```python
from build123d import *

# Parameters (mm, degrees)
F0_R     = 37
F1_DEPTH = 10
F2_R     = 37
F3_DEPTH = 75
F4_R     = 37
F4_R_2   = 30
F4_W     = 13
F4_H     = 13
F5_DEPTH = 10


with BuildPart() as f1:
    # F0 (on Top) → F1 (new body)
    with BuildSketch(Plane.XY):
        Circle(F0_R)
        with BuildLine():
            ThreePointArc((32.403703492, 2.5), (32.47591695, 1.250926958), (32.5, 0))
            ThreePointArc((32.5, 0), (32.47591695, -1.250926958), (32.403703492, -2.5))
            ThreePointArc((32.403703492, -2.5), (22.9809703886, -22.9809703886), (2.5, -32.403703492))
            ThreePointArc((2.5, -32.403703492), (0, -32.5), (-2.5, -32.403703492))
            ThreePointArc((-2.5, -32.403703492), (-22.9809703886, -22.9809703886), (-32.403703492, -2.5))
            ThreePointArc((-32.403703492, -2.5), (-32.5, 0), (-32.403703492, 2.5))
            ThreePointArc((-32.403703492, 2.5), (-22.9809703886, 22.9809703886), (-2.5, 32.403703492))
            ThreePointArc((-2.5, 32.403703492), (0, 32.5), (2.5, 32.403703492))
            ThreePointArc((2.5, 32.403703492), (22.9809703886, 22.9809703886), (32.403703492, 2.5))
        make_face(mode=Mode.SUBTRACT)
        with BuildLine():
            Line((2.5, 29.5), (2.5, 32.403703492))
            ThreePointArc((2.5, 32.403703492), (0, 32.5), (-2.5, 32.403703492))
            Line((-2.5, 32.403703492), (-2.5, 29.5))
            Line((-2.5, 29.5), (2.5, 29.5))
        make_face()
        with BuildLine():
            ThreePointArc((32.403703492, -2.5), (32.47591695, -1.250926958), (32.5, 0))
            ThreePointArc((32.5, 0), (32.47591695, 1.250926958), (32.403703492, 2.5))
            Line((32.403703492, 2.5), (29.5, 2.5))
            Line((29.5, 2.5), (29.5, -2.5))
            Line((29.5, -2.5), (32.403703492, -2.5))
        make_face()
        with BuildLine():
            ThreePointArc((-2.5, -32.403703492), (0, -32.5), (2.5, -32.403703492))
            Line((2.5, -32.403703492), (2.5, -29.5))
            Line((2.5, -29.5), (-2.5, -29.5))
            Line((-2.5, -29.5), (-2.5, -32.403703492))
        make_face()
        with BuildLine():
            Line((-29.5, 2.5), (-32.403703492, 2.5))
            ThreePointArc((-32.403703492, 2.5), (-32.5, 0), (-32.403703492, -2.5))
            Line((-32.403703492, -2.5), (-29.5, -2.5))
            Line((-29.5, -2.5), (-29.5, 2.5))
        make_face()
    extrude(amount=-F1_DEPTH)

    # F2 (on face) → F3 (join)
    with BuildSketch(Plane(origin=(0, 0, -10), x_dir=(1, 0, 0), z_dir=(0, 0, -1))):
        Circle(F2_R)
        with BuildLine():
            ThreePointArc((29.8956518578, 2.5), (29.9739016123, 1.2510883797), (30, 0))
            ThreePointArc((30, 0), (29.9739016123, -1.2510883797), (29.8956518578, -2.5))
            Line((29.8956518578, -2.5), (32.403703492, -2.5))
            ThreePointArc((32.403703492, -2.5), (22.9809703886, -22.9809703886), (2.5, -32.403703492))
            Line((2.5, -32.403703492), (2.5, -29.8956518578))
            ThreePointArc((2.5, -29.8956518578), (0, -30), (-2.5, -29.8956518578))
            Line((-2.5, -29.8956518578), (-2.5, -32.403703492))
            ThreePointArc((-2.5, -32.403703492), (-22.9809703886, -22.9809703886), (-32.403703492, -2.5))
            Line((-32.403703492, -2.5), (-29.8956518578, -2.5))
            ThreePointArc((-29.8956518578, -2.5), (-30, 0), (-29.8956518578, 2.5))
            Line((-29.8956518578, 2.5), (-32.403703492, 2.5))
            ThreePointArc((-32.403703492, 2.5), (-22.9809703886, 22.9809703886), (-2.5, 32.403703492))
            Line((-2.5, 32.403703492), (-2.5, 29.8956518578))
            ThreePointArc((-2.5, 29.8956518578), (0, 30), (2.5, 29.8956518578))
            Line((2.5, 29.8956518578), (2.5, 32.403703492))
            ThreePointArc((2.5, 32.403703492), (22.9809703886, 22.9809703886), (32.403703492, 2.5))
            Line((32.403703492, 2.5), (29.8956518578, 2.5))
        make_face(mode=Mode.SUBTRACT)
        with BuildLine():
            Line((32.403703492, -2.5), (29.8956518578, -2.5))
            ThreePointArc((29.8956518578, -2.5), (21.2132034356, -21.2132034356), (2.5, -29.8956518578))
            Line((2.5, -29.8956518578), (2.5, -32.403703492))
            ThreePointArc((2.5, -32.403703492), (22.9809703886, -22.9809703886), (32.403703492, -2.5))
        make_face()
        with BuildLine():
            Line((-2.5, -32.403703492), (-2.5, -29.8956518578))
            ThreePointArc((-2.5, -29.8956518578), (-21.2132034356, -21.2132034356), (-29.8956518578, -2.5))
            Line((-29.8956518578, -2.5), (-32.403703492, -2.5))
            ThreePointArc((-32.403703492, -2.5), (-22.9809703886, -22.9809703886), (-2.5, -32.403703492))
        make_face()
        with BuildLine():
            ThreePointArc((-29.8956518578, 2.5), (-21.2132034356, 21.2132034356), (-2.5, 29.8956518578))
            Line((-2.5, 29.8956518578), (-2.5, 32.403703492))
            ThreePointArc((-2.5, 32.403703492), (-22.9809703886, 22.9809703886), (-32.403703492, 2.5))
            Line((-32.403703492, 2.5), (-29.8956518578, 2.5))
        make_face()
        with BuildLine():
            ThreePointArc((2.5, 29.8956518578), (21.2132034356, 21.2132034356), (29.8956518578, 2.5))
            Line((29.8956518578, 2.5), (32.403703492, 2.5))
            ThreePointArc((32.403703492, 2.5), (22.9809703886, 22.9809703886), (2.5, 32.403703492))
            Line((2.5, 32.403703492), (2.5, 29.8956518578))
        make_face()
    extrude(amount=F3_DEPTH)

    # F4 (on face) → F5 (join)
    with BuildSketch(Plane(origin=(0, 0, -85), x_dir=(1, 0, 0), z_dir=(0, 0, -1))):
        Circle(F4_R)
        Circle(F4_R_2, mode=Mode.SUBTRACT)
        Circle(F4_R_2)
        Rectangle(F4_W, F4_H, mode=Mode.SUBTRACT)
    extrude(amount=F5_DEPTH)


solid = f1.part
```
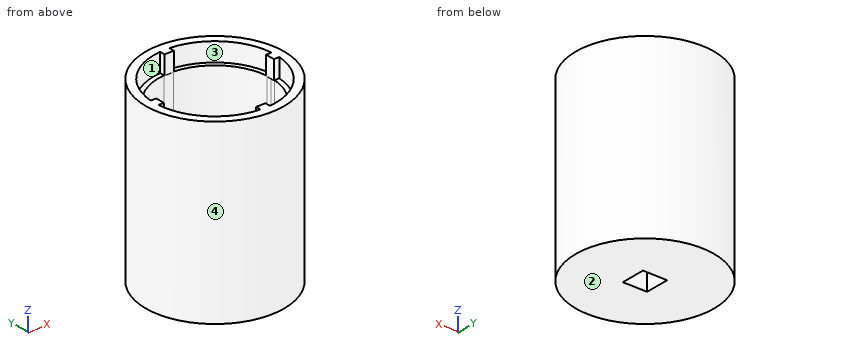
Here's how the part is built. I have some questions about the finished solid (model axes, mm). Face numbers are marked on the shaded views. Give positions to 0.01 mm unless a question says otherwise; leave off trailing zeros. Loops run counter-clockwise (first coordinate to the right, second up) from the corner with the lowest first, then second, coordinate; pieces in that order, holes last. Notation, with made-up numbers: M 38,-9 L 94,-9 A23 ccw 94,22 Z; hole C 45,51.25 d6. An arc over 180 degrees is marked long. Return JSON: item names as keys, results as strings.
Item 1: Imagine slicing it at D-D on x = -9.5. List the corners of the cut face in (y, z) for me.
A:
{"outline": "M -35.76,-95 L 35.76,-95 L 35.76,0 L 31.08,0 L 31.08,-10 L 28.46,-10 L 28.46,-85 L -28.46,-85 L -28.46,-10 L -31.08,-10 L -31.08,0 L -35.76,0 Z"}
Item 2: Imagine slicing it at A-A on x = 0. List the corners of the cut face in (y, z) for me.
A:
{"outline": "M -37,-95 L -6.5,-95 L -6.5,-85 L -30,-85 L -30,-10 L -29.5,-10 L -29.5,0 L -37,0 Z; M 6.5,-95 L 37,-95 L 37,0 L 29.5,0 L 29.5,-10 L 30,-10 L 30,-85 L 6.5,-85 Z"}
Item 3: Imagine slicing it at B-B on z = -53. List the corners of the cut face in (x, y) for me, then the cut area to 3 significant figures.
A:
{"outline": "C 0,0 d74; hole C 0,0 d60", "area": "1,470 mm^2"}
Item 4: Imagine slicing it at C-C on x = -18.5. List the corners of the cut face in (y, z) for me, then the cut area to 3 significant figures.
A:
{"outline": "M -32.04,-95 L 32.04,-95 L 32.04,0 L 26.72,0 L 26.72,-10 L 23.62,-10 L 23.62,-85 L -23.62,-85 L -23.62,-10 L -26.72,-10 L -26.72,0 L -32.04,0 Z", "area": "2,010 mm^2"}
Item 5: Thinking about a two-plate mould opening in X: for the marked faces 1, 2, 3 and 4, which applies, released by +X, released by -X, zero draft, split by the parting line, or undercut?
A:
{"face 1": "undercut", "face 2": "zero draft", "face 3": "undercut", "face 4": "split by the parting line"}
Item 6: Please list where these lines run through material, in increasing order: line 1 (X direction, y = 1, z = -16.5); line 2 (Y direction, x = 0.5, z = -9); line 3 (Z direction, x = -23.5, y = -10.5).
A:
{"line 1": "x = -36.99 to -29.98, 29.98 to 36.99", "line 2": "y = -37 to -29.5, 29.5 to 37", "line 3": "z = -95 to -85"}
Item 7: I'm going to push flat-ended pins straight in: pin 1 Ø1.5 at (x, z) = (-1, -5) entering from -Y; pin 2 Ø8 at (x, z) = (-6, -84) entering from +Y; pin 3 Ø2.5 at (x, z) = (0, -3.5) entering from +Y; pin 4 Ø15 at (x, y) = (17.5, 24.5) entering from +Z. Where does each tip first touch, or does it pass through?
A:
{"pin 1": "stops at y = -37", "pin 2": "stops at y = 36.95", "pin 3": "stops at y = 37", "pin 4": "stops at z = 0"}
